The model under review builds one solid part; all positions refer to its coordinate system, in mm. Round coordinates to 2 decimals unless told otherwise and drop trailing zeros. Loops run counter-clockwise (first coordinate to the right, second up) from the corner with the lowest first, then second, coordinate; pieces in that order, holes last. Notation, with made-up numbers: M 9,58 L 31,58 A19 cw 31,79 Z; hole C 66.5,-24.75 d3. An arc over 180 degrees is marked long. Use a Markdown table: item, result. Add a question column.
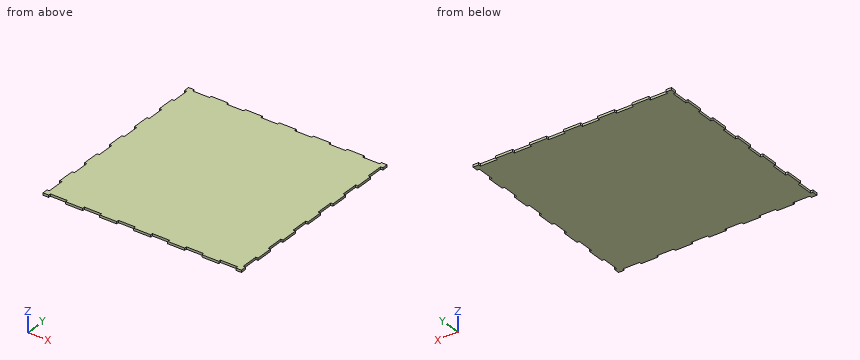
Autodesk Fusion 360 part; units mm, degrees
sketch "Sketch1" plane through (0, 0, 0) normal (0, 0, 1) x (1, 0, 0)
  line L0 (0, 0) -> (350, 0)
  line L1 (350, 0) -> (350, 350)
  line L2 (350, 350) -> (0, 350)
  line L3 (0, 350) -> (0, 0)
  point P0 (175, 175)
  dimension "d1" = 350
  dimension "d2" = 350
  dimension "d7" = 175
  dimension "d8" = 175
extrude "Extrude1" add sketch "Sketch1" along normal blind 4 makes body 1
sketch "Sketch2" plane through (0, 0, 4) normal (0, 0, 1) x (-1, 0, 0)
  line L0 (0, -350) -> (0, 0)
  line L1 (-10, 0) -> (-40, 0)
  line L2 (-40, 0) -> (-40, -4)
  line L3 (-40, -4) -> (-10, -4)
  line L4 (-10, -4) -> (-10, 0)
  line L5 (0, -10) -> (-4, -10)
  line L6 (-4, -10) -> (-4, -40)
  line L7 (-4, -40) -> (0, -40)
  line L8 (0, -40) -> (0, -10)
  line L9 (0, 0) -> (-350, 0)
  dimension "d12" = 10
  dimension "d14" = 30
  dimension "d15" = 4
  dimension "d26" = 30
  dimension "d27" = 4
  dimension "d47" = 10
extrude "Extrude4" cut sketch "Sketch2" against normal through all contours L0 L5 L6 L7 L8 bodies 1
extrude "Extrude5" cut sketch "Sketch2" against normal through all contours L1 L2 L3 L4 L9 bodies 1
pattern_linear "R-Pattern1" count 6 spacing 60 along (0, 1, 0) count 2 spacing 346 along (1, 0, 0) of "Extrude4"
pattern_linear "R-Pattern2" count 6 spacing 60 along (1, 0, 0) count 2 spacing 346 along (0, 1, 0) of "Extrude5"
copy_body "Body->Comp1" bodies 1 removing the originals makes body 2 in component "Component"
component "Component" placed x (1, 0, 0) y (0, 1, 0) z (0, 0, 1) at (0, 0, 0)
equation "d1 = Linear Dimension-2"
equation "d2 = Linear Dimension-3"
equation "d7 = d / 2"
equation "d8 = b / 2"
equation "d12 = b_corner"
equation "b_corner = ( b - ( floor(b / a) * a ) ) / 2"
equation "d14 = Linear Dimension-3"
equation "d15 = Linear Dimension-4"
equation "d26 = Linear Dimension-5"
equation "d27 = Linear Dimension-6"
equation "d_corner = ( d - ( floor(d / a) * a ) ) / 2"
equation "d41 = 2 * a"
equation "d42 = b - t"
equation "d45 = 2 * a"
equation "d46 = d - t"
equation "d47 = d_corner"
(1) To check wall thickness, follow probe 1 along X at (y, z) = (260, 0.8). State the ranges of the line that lie inside material, in increasing order.
(2) Insertion check: pin 1 Ø1.2 at (x, z) = (2, 2.5) entering from -Y; pin 2 Ø1.5 at (y, z) = (93.5, 2.5) entering from -X. Each pin has a flat end and moves straight along its axis. Give the tip position at first contact, or say it passes through.
(3) Consider section A-A, the plane y = 88. Give the boundary of the cut face in (x, z).
Found:
| question | item | result |
|---|---|---|
| 1 | probe 1 | x = 4 to 346 |
| 2 | pin 1 | stops at y = 0 |
| 2 | pin 2 | stops at x = 4 |
| 3 | outline | M 4,0 L 346,0 L 346,4 L 4,4 Z |
